The figure shows three views and two pictorial views of one solid part (mm, origin at its lowest corner). Answer the questions. A direction names the side the tool comes from. Round coordinates to 2 decimals unless told otherwise and drop trailing zeros. Write each loop counter-clockwise with the first axis right and the second up, starting at its lowest first coordinate (ties: lowest second). Pieces come first, ordered by that corner, then holes. Notation, with made-up numbers: (44.25, 37) -> (54.25, 37) arc R8 cw to (54.25, 51) -> close; hole circle Ø1 at (-4.75, -17). An arc over 180 degrees is marked (long way). One line per item, written item: value.
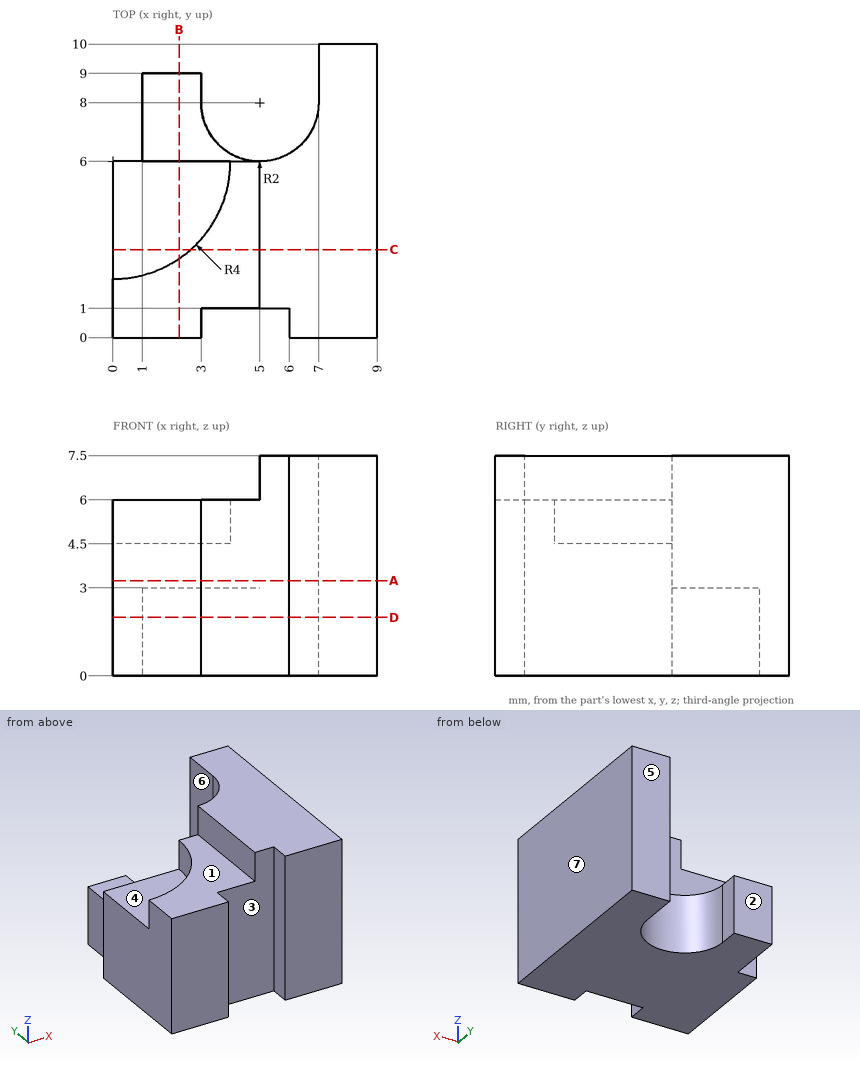
(1) Flat-ended cylindrical pins translate along their axes: pin 1 Ø2.5 at (x, y) = (3.5, 4) entering from +Z; pin 2 Ø1.5 at (x, y) = (2, 8) entering from +Z; pin 3 Ø2.5 at (x, z) = (2, 1.5) entering from +Y. Find the tip coordinate at first contact, or state that the pin passes through.
Reported:
pin 1: stops at z = 6
pin 2: stops at z = 3
pin 3: stops at y = 9
(2) Find section B-B on x = 2.25. Give the vertices of the cut face in (y, z), plus the area to 3 significant figures.
Reported:
outline: (0, 0) -> (9, 0) -> (9, 3) -> (6, 3) -> (6, 4.5) -> (2.69, 4.5) -> (2.69, 6) -> (0, 6) -> close
area: 40.0 mm2
(3) Find section A-A on z = 3.25. Give the vertices of the cut face in (x, y), plus the area to 3 significant figures.
Reported:
outline: (0, 0) -> (3, 0) -> (3, 1) -> (6, 1) -> (6, 0) -> (9, 0) -> (9, 10) -> (7, 10) -> (7, 8) arc R2 cw to (5, 6) -> (0, 6) -> close
area: 59.9 mm2
(4) For a pull along X with two mould halves and no side action, classify the marked faces 5, 6 and 7 as pulls with the +X half, pulls with the -X half, needs draft (parallel to the pull), parting line crosses it, or undercut.
Reported:
face 5: needs draft
face 6: undercut
face 7: pulls with the +X half
(5) Find section C-C on y = 3. Give the vertices of the cut face in (x, z).
Reported:
outline: (0, 0) -> (9, 0) -> (9, 7.5) -> (5, 7.5) -> (5, 6) -> (2.65, 6) -> (2.65, 4.5) -> (0, 4.5) -> close
(6) A tool of negligible diameter and unlimited length cuts with its end or side. For the marked faces 1, 2, 3 and 4, from which of +Z, -Z, +X, -X, +Y, -Y can it reach the whole face along a straight path? Write none if from no direction.
Reported:
face 1: +Z, -X, +Y, -Y
face 2: +Z, -Z, -X, +Y
face 3: +Z, -Z, -Y
face 4: +Z, -X, +Y
(7) Consider probe 1 along X at (y, z) = (0.75, 3.5); probe 2 along X at (y, z) = (9.5, 2.5); probe 3 along Z at (x, y) = (2, 8.25). Determine where each line is inside the solid, lowest interval first.
Reported:
probe 1: x = 0 to 3, 6 to 9
probe 2: x = 7 to 9
probe 3: z = 0 to 3
(8) Find section D-D on z = 2. Give the vertices of the cut face in (x, y), plus the area to 3 significant figures.
Reported:
outline: (0, 0) -> (3, 0) -> (3, 1) -> (6, 1) -> (6, 0) -> (9, 0) -> (9, 10) -> (7, 10) -> (7, 8) arc R2 cw to (3, 8) -> (3, 9) -> (1, 9) -> (1, 6) -> (0, 6) -> close
area: 66.7 mm2
